Autodesk Inventor part; units mm, degrees
ref_plane "Plan de construction1" through (-63.7723, 27.6488, 10.9) normal (0, 0, 1) x (1, 0, 0)
ref_plane "YZ Plane" through (0, 0, 0) normal (1, 0, 0) x (0, 1, 0)
ref_plane "XZ Plane" through (0, 0, 0) normal (0, 1, 0) x (-1, 0, 0)
sketch "Esquisse1" plane through (0, 0, 0) normal (0, 0, 1) x (1, 0, 0)
  line L0 (-73.2723, 18.1488) -> (-54.2723, 18.1488)
  line L1 (-54.2723, 18.1488) -> (-54.2723, 37.1488)
  line L2 (-54.2723, 37.1488) -> (-73.2723, 37.1488)
  line L3 (-73.2723, 37.1488) -> (-73.2723, 18.1488)
  circle A0 centre (-63.7723, 27.6488) radius 4.5
  point P0 (0, 0)
  dimension "d0" = 19
  dimension "d1" = 19
  dimension "d2" = 9
extrude "Extrusion1" add sketch "Esquisse1" along normal blind 10
sketch "Esquisse2" plane through (-73.2723, 37.1488, 0) normal (0, 1, 0) x (1, 0, 0)
  line L0 (0, 0) -> (0, -10)
  line L1 (19, 0) -> (19, -10)
  line L2 (19, -10) -> (0, -10)
  point P0 (73.2723, 0)
  point P1 (2, -5)
  point P2 (17, -5)
  dimension "d5" = 2
  dimension "d6" = 2
  dimension "d7" = 5
  dimension "d8" = 5
hole "Perçage1" at (-71.2723, 37.1488, 5) at (-56.2723, 37.1488, 5) direction (0, -1, 0) diameter 2 end through all
ref_plane "Plan de construction1" through (-63.7723, 27.6488, 10.9) normal (0, 0, 1) x (1, 0, 0)
properties part number "palier_roulement_bras"
For this review, take the finished solid that the model builds, in its own axes (mm). Coordinates: 2 decimals unless noted, no trailing zeros. Write each loop counter-clockwise with the first axis right and the second up, starting at its lowest first coordinate (ties: lowest second). Pieces come first, ordered by that corner, then holes. Notation, with made-up numbers: (63, 31.25) -> (94, 31.25) arc R31 cw to (94, 61.25) -> close; hole circle Ø5 at (40.5, 4.5). An arc over 180 degrees is marked (long way). Write each question's results on one line, items separated by ' | '. Start each with the question number.
1) Consider section C-C (y = 23.5). Write out the cut boundary in (x, z), plus the area to 3 significant figures.
2) The part is to be moulded in two halves that separate along X. For faces 1 (the face through (-54.272, 28, 5)), 2 (the face through (-64, 37.149, 5)), 3 (the face through (-72.264, 27.516, 4.87)), say which applies: +X half, -X half, draft (parallel to the pull), parting line (faces both ways), or undercut.
3) Insertion check: pin 1 (8 mm diameter, centred on x = -63.77, y = 27.65, fed in from +Z); pin 2 (2.5 mm diameter, centred on x = -56.27, z = 5, fed in from -Y). Each pin has a flat end and moves straight along its axis. Give the tip position at first contact, or say it passes through.
4) Consider section A-A (y = 30.75). Write out the cut boundary in (x, z), plus the area to 3 significant figures.
5) Consider section B-B (z = 5). Write out the cut boundary in (x, y), plus the area to 3 significant figures.
6) Wall thickness on L1, parallel to X at y = 22.25, z = 5; L2, parallel to X at y = 27, z = 5; L3, parallel to X at y = 35.25, z = 4.25: over which ranges is each line inside the solid? List them lowest first. Write a range as [from, to].
7) Consider section D-D (z = 3.75). Write out the cut boundary in (x, y), plus the area to 3 significant figures.
Geometry says:
1) outline: (-73.27, 0) -> (-65.52, 0) -> (-65.52, 10) -> (-73.27, 10) -> close; (-62.03, 0) -> (-54.27, 0) -> (-54.27, 10) -> (-62.03, 10) -> close; hole circle Ø2 at (-71.27, 5); hole circle Ø2 at (-56.27, 5) | area: 149 mm^2
2) face 1: +X half | face 2: draft | face 3: undercut
3) pin 1: through | pin 2: y = 18.15
4) outline: (-73.27, 0) -> (-67.03, 0) -> (-67.03, 10) -> (-73.27, 10) -> close; (-60.51, 0) -> (-54.27, 0) -> (-54.27, 10) -> (-60.51, 10) -> close; hole circle Ø2 at (-71.27, 5); hole circle Ø2 at (-56.27, 5) | area: 119 mm^2
5) outline: (-73.27, 18.15) -> (-72.27, 18.15) -> (-72.27, 37.15) -> (-73.27, 37.15) -> close; (-70.27, 18.15) -> (-57.27, 18.15) -> (-57.27, 37.15) -> (-70.27, 37.15) -> close; (-55.27, 18.15) -> (-54.27, 18.15) -> (-54.27, 37.15) -> (-55.27, 37.15) -> close; hole circle Ø9 at (-63.77, 27.65) | area: 221 mm^2
6) L1: [-73.27, -72.27], [-70.27, -57.27], [-55.27, -54.27] | L2: [-73.27, -72.27], [-70.27, -68.23], [-59.32, -57.27], [-55.27, -54.27] | L3: [-73.27, -71.93], [-70.61, -56.93], [-55.61, -54.27]
7) outline: (-73.27, 18.15) -> (-54.27, 18.15) -> (-54.27, 37.15) -> (-73.27, 37.15) -> close; hole circle Ø9 at (-63.77, 27.65) | area: 297 mm^2
